CAD build for the part. Positions are in the model's coordinates, mm. Face numbers are marked on the shaded views. Round coordinates to 2 decimals unless told otherwise and drop trailing zeros. Write each loop counter-clockwise with the first axis right and the second up, starting at its lowest first coordinate (ties: lowest second). Pieces come first, ordered by that corner, then holes. Notation, with made-up numbers: (-15, 35.25) - (35, 35.25) arc R28 cw to (35, 60.25) - close; hole circle Ø11 at (-7, 24). An arc over 180 degrees is marked (long way). Use one line per item in the form item = value. Start each with the question number.
Item 1: Pull direction Y, two halves, no side cores. Call the marked faces 1, 2, 3 and 4: +Y half, -Y half, draft (parallel to the pull), parting line (faces both ways), or undercut.
Item 2: Pin check, flat tips, straight feed: pin 1 (8 mm diameter, centred on x = 26.5, y = 37, fed in from +Z); pin 2 (1.8 mm diameter, centred on y = 25, z = 1.5, fed in from +X). Stop position of each tip, or through.
Item 3: Band-saw the part on D-D, the plane y = 4. List the corners of the cut face in (x, z).
Item 4: Band-saw the part on A-A, the plane z = 10.25. List the corners of the cut face in (x, y).
Item 5: Band-saw the part on C-C, the plane x = -26. List the corners of the cut face in (y, z).
Item 6: Band-saw the part on B-B, the plane y = -54. List the corners of the cut face in (x, z).
Item 7: Drill centre lines: L1, parallel to Y at x = -53.5, z = 8.5; L2, parallel to X at y = -28, z = 9.75; L3, parallel to Y at x = 57.5, z = 0.75. Where is each one in solid material? Low to high.
from build123d import *

# Parameters (mm, degrees)
SKETCH1_W           = 34
SKETCH1_H           = 34
BOSS_EXTRUDE1_DEPTH = 6
BOSS_EXTRUDE2_DEPTH = 6


with BuildPart() as part:
    # Sketch1 → Boss-Extrude1 (new body)
    # profile 1 of 4: a face of its own
    with BuildSketch(Plane.XY):
        Polygon((64, 21.972155185), (55.873, 17.280029547), (55.873, 32.719970453), (64, 28.027844815), (64, 65), (-64, 65), (-64, -65), (64, -65), (64, -28.027844815), (55.873, -32.719970453), (55.873, -17.280029547), (64, -21.972155185), align=None)
        with Locations((32, 0)):
            Rectangle(SKETCH1_W, SKETCH1_H, mode=Mode.SUBTRACT)
        with Locations((32, -40)):
            Rectangle(SKETCH1_W, SKETCH1_H, mode=Mode.SUBTRACT)
        with Locations((32, 40)):
            Rectangle(SKETCH1_W, SKETCH1_H, mode=Mode.SUBTRACT)
    # profile 2 of 4: a face of its own
    with BuildSketch(Plane.XY):
        with Locations((32, 0)):
            Rectangle(SKETCH1_W, SKETCH1_H)
    # profile 3 of 4: a face of its own
    with BuildSketch(Plane.XY):
        with Locations((32, 40)):
            Rectangle(SKETCH1_W, SKETCH1_H)
    # profile 4 of 4: a face of its own
    with BuildSketch(Plane.XY):
        with Locations((32, -40)):
            Rectangle(SKETCH1_W, SKETCH1_H)
    extrude(amount=BOSS_EXTRUDE1_DEPTH)

    # Sketch2 → Boss-Extrude2 (add)
    with BuildSketch(Plane.XY.offset(6)):
        Polygon((-64, 65), (64, 65), (64, 15), (54, 15), (54, 59), (-58, 59), (-58, -59), (54, -59), (54, -15), (64, -15), (64, -65), (-64, -65), align=None)
    extrude(amount=BOSS_EXTRUDE2_DEPTH)


solid = part.part
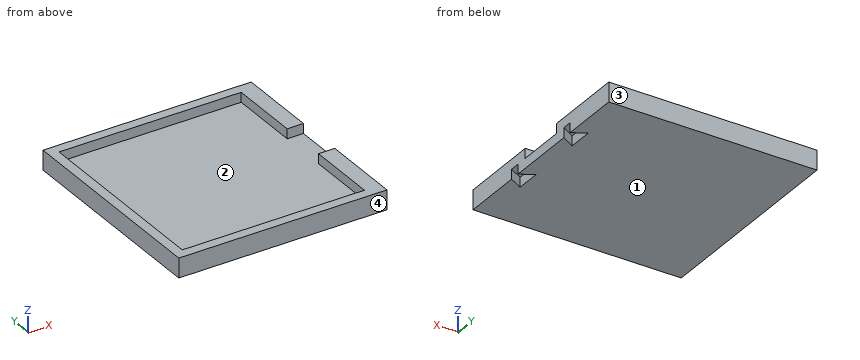
Determined:
q1.face_1 = draft
q1.face_2 = undercut
q1.face_3 = +Y half
q1.face_4 = -Y half
q2.pin_1 = 6
q2.pin_2 = 55.87
q3.outline = (-64, 0) - (64, 0) - (64, 6) - (-58, 6) - (-58, 12) - (-64, 12) - close
q4.outline = (-64, -65) - (64, -65) - (64, -15) - (54, -15) - (54, -59) - (-58, -59) - (-58, 59) - (54, 59) - (54, 15) - (64, 15) - (64, 65) - (-64, 65) - close
q5.outline = (-65, 0) - (65, 0) - (65, 12) - (59, 12) - (59, 6) - (-59, 6) - (-59, 12) - (-65, 12) - close
q6.outline = (-64, 0) - (64, 0) - (64, 12) - (54, 12) - (54, 6) - (-58, 6) - (-58, 12) - (-64, 12) - close
q7.L1 = -65 to -59, 59 to 65
q7.L2 = -64 to -58, 54 to 64
q7.L3 = -65 to -31.78, -18.22 to 18.22, 31.78 to 65
